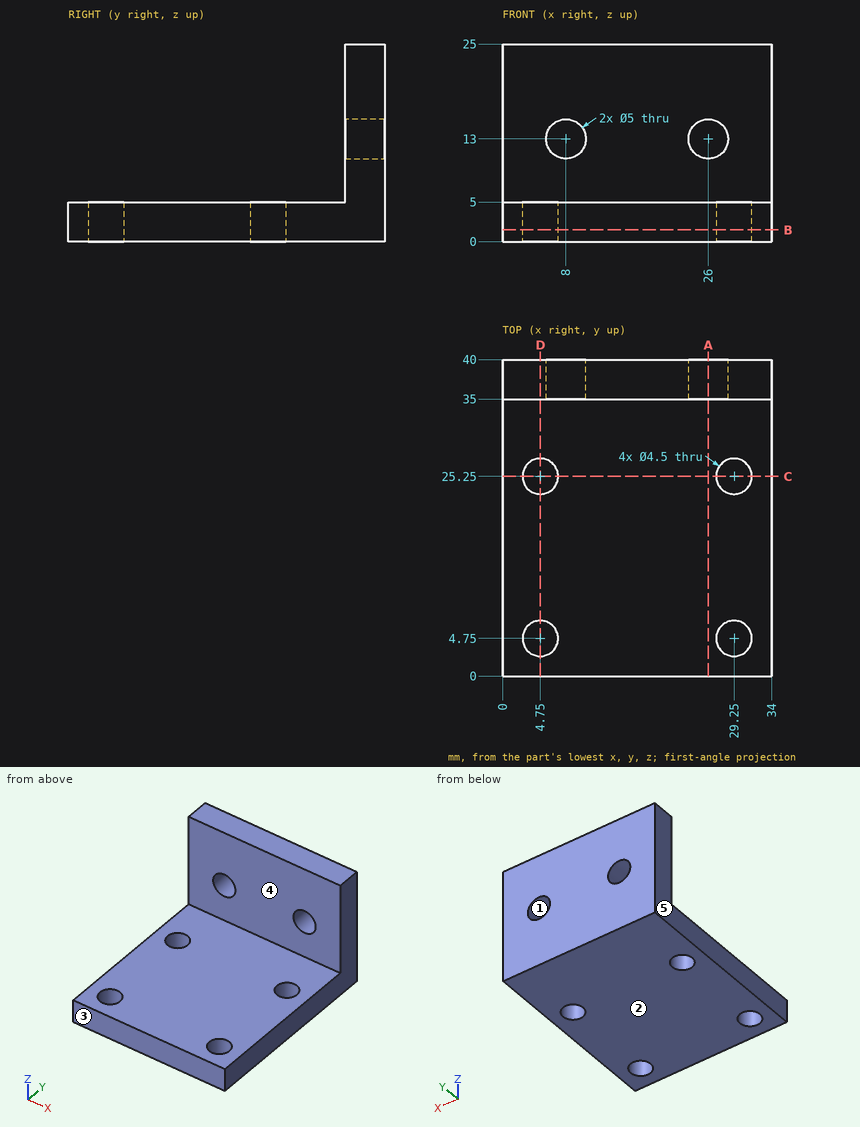
Design review of the part shown in the three views and the two pictorial views. Dimensions are in mm from the part's minimum x, y and z. A direction names the side the tool comes from. Round coordinates to 2 decimals unless told otherwise and drop trailing zeros. Write each loop counter-clockwise with the first axis right and the second up, starting at its lowest first coordinate (ties: lowest second). Pieces come first, ordered by that corner, then holes.
Item 1: Wall thickness on L1, parallel to X at y = 38.25, z = 13; L2, parallel to Y at x = 29.25, z = 1.15; L3, parallel to Z at x = 33, y = 16: over which ranges is each line inside the solid? List them lowest first.
Item 2: Consider section D-D on x = 4.75. Give the boundary of the cut face in (y, z), and give its area (3 significant figures).
Item 3: Draft analysis for pull direction Z (two halves, no side actions). For the marked faces 1, 2 and 3, state which applies: released by +Z, released by -Z, zero draft, split by the parting line, or undercut.
Item 4: Consider section C-C on y = 25.25. Give the boundary of the cut face in (x, z).
Item 5: For pin 1 Ø1.5 at (y, z) = (11.5, 4) entering from -X; pin 2 Ø5 at (x, y) = (29.25, 25.25) entering from +Z; pin 3 Ø10 at (x, z) = (17, 14) entering from -Y, all flat-tipped, find the tip position at first contact; note any pin that passes through.
Item 6: Consider section A-A on x = 26. Give the boundary of the cut face in (y, z), and give its area (3 significant figures).
Item 7: Consider section B-B on z = 1.5. Give the boundary of the cut face in (x, y), and give its area (3 significant figures).
Item 8: For the marked faces 4 and 5, list the 3-axis set-ups (+Z, -Z, +X, -X, +Y, -Y) from which the entire face can be reached by the end or side of a thin tool; tool diameter is ignored.
Check values:
1. L1: x = 0 to 5.5, 10.5 to 23.5, 28.5 to 34
1. L2: y = 0 to 2.5, 7 to 23, 27.5 to 40
1. L3: z = 0 to 5
2. outline: (0, 0) - (2.5, 0) - (2.5, 5) - (0, 5) - close; (7, 0) - (23, 0) - (23, 5) - (7, 5) - close; (27.5, 0) - (40, 0) - (40, 25) - (35, 25) - (35, 5) - (27.5, 5) - close
2. area: 255 mm2
3. face 1: undercut
3. face 2: released by -Z
3. face 3: zero draft
4. outline: (0, 0) - (2.5, 0) - (2.5, 5) - (0, 5) - close; (7, 0) - (27, 0) - (27, 5) - (7, 5) - close; (31.5, 0) - (34, 0) - (34, 5) - (31.5, 5) - close
5. pin 1: stops at x = 0
5. pin 2: stops at z = 5
5. pin 3: stops at y = 35
6. outline: (0, 0) - (40, 0) - (40, 10.5) - (35, 10.5) - (35, 5) - (0, 5) - close; (35, 15.5) - (40, 15.5) - (40, 25) - (35, 25) - close
6. area: 275 mm2
7. outline: (0, 0) - (34, 0) - (34, 40) - (0, 40) - close; hole circle Ø4.5 at (4.75, 4.75); hole circle Ø4.5 at (4.75, 25.25); hole circle Ø4.5 at (29.25, 4.75); hole circle Ø4.5 at (29.25, 25.25)
7. area: 1,300 mm2
8. face 4: +Z, +X, -X, -Y
8. face 5: +Z, -Z, -X, +Y, -Y
